Here's how the part is built. I have some questions about the finished solid (model axes, mm). A direction names the side the tool comes from. Coordinates: 2 decimals unless noted, no trailing zeros. Order: outer loops, then holes, each group sorted by start corner. A loop starts at its lowest first (then second) coordinate and runs counter-clockwise, first axis right, second up. Notation, with made-up numbers: (39, 1.25) - (54, 1.25) arc R10 ccw to (54, 13.25) - close; hole circle Ø1 at (76.25, 51.25). An arc over 180 degrees is marked (long way). Use CSV: the item, a comma, the result in double quotes. Start each with the question number.
from build123d import *

# Parameters (mm, degrees)
CROQUIS1_R                    = 6
SALIENTE_EXTRUIR1_DEPTH       = 6
CROQUIS2_R                    = 7.25
SALIENTE_EXTRUIR2_DEPTH       = 0.5
CROQUIS3_R                    = 11.5
SALIENTE_EXTRUIR3_DEPTH       = 1.2
CROQUIS4_R                    = 9.125
SALIENTE_EXTRUIR4_DEPTH       = 11.6
CROQUIS5_R                    = 11.5
SALIENTE_EXTRUIR5_DEPTH       = 1.2
CROQUIS6_R                    = 7.25
SALIENTE_EXTRUIR6_DEPTH       = 0.5
CROQUIS7_R                    = 4
CORTAR_EXTRUIR1_DEPTH         = 27.561249971
TALADRO_ROSCADO_M32_D         = 2.5
TALADRO_ROSCADO_M32_DEPTH     = 8.5
TALADRO_ROSCADO_M32_TIP       = 0.751075774
TALADRO_ROSCADO_M33_OUTLINE_W = 1.25
TALADRO_ROSCADO_M33_OUTLINE_H = 5.325356109


# Read off the part's stored shape, not the designer's step: Taladro roscado M33
with BuildPart() as part:
    # Croquis1 → Saliente-Extruir1 (new body)
    with BuildSketch(Plane(origin=(0, 0, 0), x_dir=(0, 0, -1), z_dir=(1, 0, 0))):
        Circle(CROQUIS1_R)
    extrude(amount=SALIENTE_EXTRUIR1_DEPTH)

    # Croquis2 → Saliente-Extruir2 (add)
    with BuildSketch(Plane(origin=(6, 0, 0), x_dir=(0, 0, -1), z_dir=(1, 0, 0))):
        Circle(CROQUIS2_R)
    extrude(amount=SALIENTE_EXTRUIR2_DEPTH)

    # Croquis3 → Saliente-Extruir3 (add)
    with BuildSketch(Plane(origin=(6.5, 0, 0), x_dir=(0, 0, -1), z_dir=(1, 0, 0))):
        Circle(CROQUIS3_R)
    extrude(amount=SALIENTE_EXTRUIR3_DEPTH)

    # Croquis4 → Saliente-Extruir4 (add)
    with BuildSketch(Plane(origin=(7.7, 0, 0), x_dir=(0, 0, -1), z_dir=(1, 0, 0))):
        Circle(CROQUIS4_R)
    extrude(amount=SALIENTE_EXTRUIR4_DEPTH)

    # Croquis5 → Saliente-Extruir5 (add)
    with BuildSketch(Plane(origin=(19.3, 0, 0), x_dir=(0, 0, -1), z_dir=(1, 0, 0))):
        Circle(CROQUIS5_R)
    extrude(amount=SALIENTE_EXTRUIR5_DEPTH)

    # Croquis6 → Saliente-Extruir6 (add)
    with BuildSketch(Plane(origin=(20.5, 0, 0), x_dir=(0, 0, -1), z_dir=(1, 0, 0))):
        Circle(CROQUIS6_R)
    extrude(amount=SALIENTE_EXTRUIR6_DEPTH)

    # Croquis7 → Cortar-Extruir1 (cut, through all)
    with BuildSketch(Plane.ZY):
        Circle(CROQUIS7_R)
    extrude(amount=-CORTAR_EXTRUIR1_DEPTH, mode=Mode.SUBTRACT)

    # Taladro roscado M32
    with Locations(Plane(origin=(0, 0, -6), x_dir=(-1, 0, 0), z_dir=(0, 0, -1))):
        with Locations((-3.5, 0)):
            Hole(TALADRO_ROSCADO_M32_D / 2, depth=TALADRO_ROSCADO_M32_DEPTH)
            with Locations((0, 0, -(TALADRO_ROSCADO_M32_DEPTH + TALADRO_ROSCADO_M32_TIP / 2))):  # 118° drill point
                Cone(0, TALADRO_ROSCADO_M32_D / 2, TALADRO_ROSCADO_M32_TIP, mode=Mode.SUBTRACT)

    # Taladro roscado M33 outline → Taladro roscado M33 (revolve, cut)
    with BuildSketch(Plane(origin=(13.5, 0, 0), x_dir=(1, 0, 0), z_dir=(0, -1, 0))):
        with Locations((0.625, -6.462322169)):
            Rectangle(TALADRO_ROSCADO_M33_OUTLINE_W, TALADRO_ROSCADO_M33_OUTLINE_H)
    revolve(axis=Axis((13.5, 0, 0), (0, 0, 1)), mode=Mode.SUBTRACT)


solid = part.part
Item 1: We'd pull the mould along Z, two halves only. Please class faces 4 (the cylindrical face through (10.353, -1.532, 3.695)), 5 (the cylindrical face through (19.9, 11.4, 1.5)), 6 (the flat face through (0, -3.92, 1.42)): released by +Z, released by -Z, zero draft, split by the parting line, or undercut.
Item 2: For pin 1 Ø3 at (x, y) = (7.5, 2.5) entering from -Z; pin 2 Ø3 at (x, y) = (3.5, 0) entering from +Z; pin 3 Ø2 at (x, y) = (13.5, 0) entering from -Z, each with a flat end and sliding along its axis, tell me the tip position at first contact or that it passes through.
Item 3: Suppose I cut it at C-C on y = -8.5. Write out the boundary of the cut face in (x, z).
Item 4: Suppose I cut it at D-D on x = 18.25. Write out the boundary of the cut face in (y, z) (3 decimals), then the cut area to 3 significant figures.
Item 5: For faces 1 (the flat face through (20.5, -8, 0)), 2 (the cylindrical face through (4.69, 0.38, -4.88)), 3 (the flat face through (19.3, 9, 3)), which set-ups out of +Z, -Z, +X, -X, +Y, -Y let a thin tool reach every point of the face, with its end or its side?
Item 6: Please list where these lines run through material, in increasing order: line 1 along X through (y, z) = (0, -5); line 2 along X through (y, z) = (10, 0.75); line 3 along Y through (x, z) = (10.25, 0) (3 decimals). Write a range as from..to.
Item 7: Suppose I cut it at B-B on y = -1.75. Write out the boundary of the cut face in (x, z), then the cut area to 3 significant figures.
Item 8: Suppose I cut it at A-A on z = 0. Write out the boundary of the cut face in (x, y) (3 decimals), then the cut area to 3 significant figures.
Here are the results:
1,face 4,"undercut"
1,face 5,"split by the parting line"
1,face 6,"zero draft"
2,pin 1,"z = -11.46"
2,pin 2,"z = 6"
2,pin 3,"z = 3.87"
3,outline,"(6.5, -7.75) - (7.7, -7.75) - (7.7, -3.32) - (19.3, -3.32) - (19.3, -7.75) - (20.5, -7.75) - (20.5, 7.75) - (19.3, 7.75) - (19.3, 3.32) - (7.7, 3.32) - (7.7, 7.75) - (6.5, 7.75) - close"
4,outline,"circle Ø18.25 at (0, 0); hole circle Ø8 at (0, 0)"
4,area,"211 mm^2"
5,face 1,"+X"
5,face 2,"-Z"
5,face 3,"none"
6,line 1,"0..2.25, 4.75..12.25, 14.75..21"
6,line 2,"6.5..7.7, 19.3..20.5"
6,line 3,"-9.125..-4, 4..9.125"
7,outline,"(0, -5.74) - (6, -5.74) - (6, -7.04) - (6.5, -7.04) - (6.5, -11.37) - (7.7, -11.37) - (7.7, -8.96) - (19.3, -8.96) - (19.3, -11.37) - (20.5, -11.37) - (20.5, -7.04) - (21, -7.04) - (21, -3.6) - (0, -3.6) - close; (0, 3.6) - (21, 3.6) - (21, 7.04) - (20.5, 7.04) - (20.5, 11.37) - (19.3, 11.37) - (19.3, 8.96) - (7.7, 8.96) - (7.7, 11.37) - (6.5, 11.37) - (6.5, 7.04) - (6, 7.04) - (6, 5.74) - (0, 5.74) - close"
7,area,"194 mm^2"
8,outline,"(0, -6) - (6, -6) - (6, -7.25) - (6.5, -7.25) - (6.5, -11.5) - (7.7, -11.5) - (7.7, -9.125) - (19.3, -9.125) - (19.3, -11.5) - (20.5, -11.5) - (20.5, -7.25) - (21, -7.25) - (21, -4) - (0, -4) - close; (0, 4) - (21, 4) - (21, 7.25) - (20.5, 7.25) - (20.5, 11.5) - (19.3, 11.5) - (19.3, 9.125) - (7.7, 9.125) - (7.7, 11.5) - (6.5, 11.5) - (6.5, 7.25) - (6, 7.25) - (6, 6) - (0, 6) - close"
8,area,"185 mm^2"
